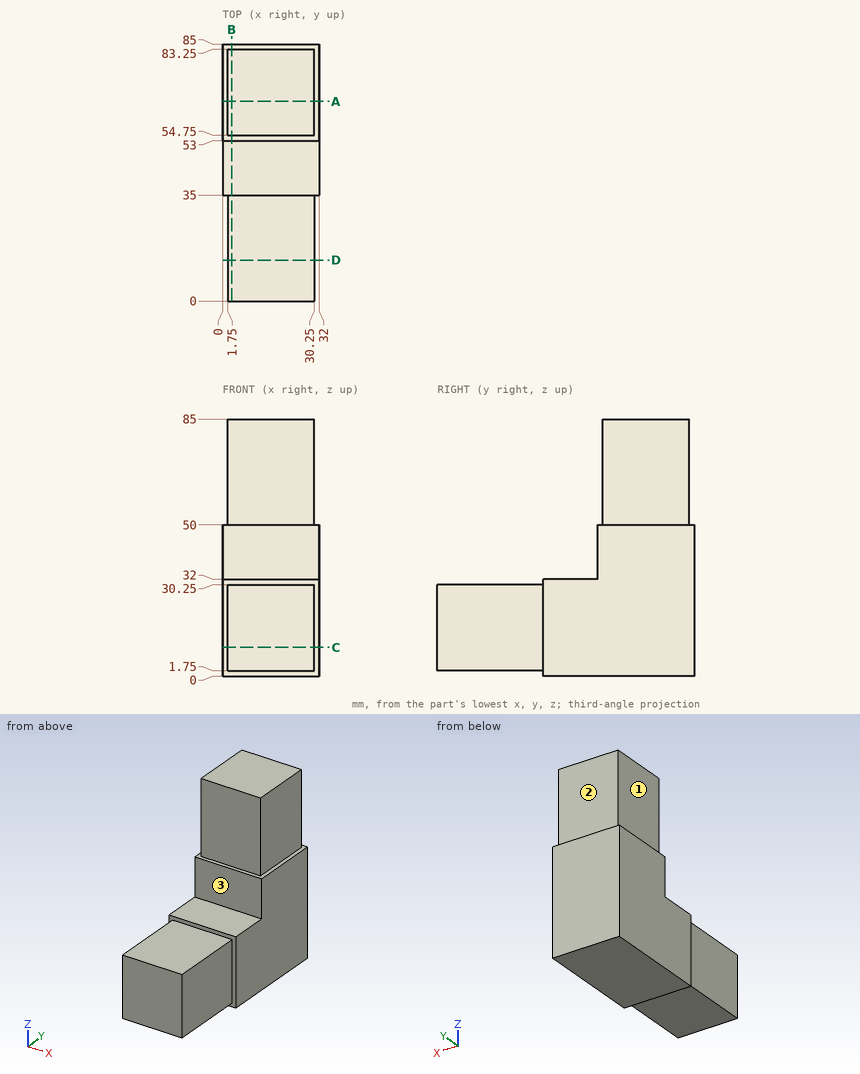
Verification items for this drawing (mm, ordinates from the low corner). A direction names the side the tool comes from. Coordinates: 2 decimals unless noted, no trailing zeros. Order: outer loops, then holes, each group sorted by start corner. A loop starts at its lowest first (then second) coordinate and runs counter-clockwise, first axis right, second up. Notation, with made-up numbers: (89.25, 57) - (130.25, 57) arc R20 ccw to (130.25, 84) - close; hole circle Ø1 at (-39.5, -13). An arc over 180 degrees is marked (long way). Use one line per item in the form item = value.
1. Access from +Z, -Z, +X, -X, +Y, -Y to the whole of each face (thin tool, end or side, straight path). Record for the marked faces 1, 2 and 3.
Here are the results:
face_1 = +Z, -X, +Y, -Y
face_2 = +Z, +X, -X, +Y
face_3 = +Z, +X, -X, -Y
2. Gauge pin test, flat ends, axial feed: pin 1 (8.5 mm diameter, centred on y = 25, z = 15.5, fed in from -X); pin 2 (9 mm diameter, centred on x = 16, z = 38.5, fed in from -Y); pin 3 (4 mm diameter, centred on x = 19, y = 45.5, fed in from +Z); pin 4 (4 mm diameter, centred on y = 36, z = 32, fed in from -X). Record the tip position at first contact, or that the pin passes through.
Here are the results:
pin_1 = 1.75
pin_2 = 53
pin_3 = 32
pin_4 = 0
3. Section check B-B (x = 3). Record the boundary of the cut face in (y, z).
Here are the results:
outline = (0, 1.75) - (35, 1.75) - (35, 0) - (85, 0) - (85, 50) - (83.25, 50) - (83.25, 85) - (54.75, 85) - (54.75, 50) - (53, 50) - (53, 32) - (35, 32) - (35, 30.25) - (0, 30.25) - close
4. Section check D-D (y = 13.5). Record the boundary of the cut face in (x, z), then the cut area to 3 significant figures.
Here are the results:
outline = (1.75, 1.75) - (30.25, 1.75) - (30.25, 30.25) - (1.75, 30.25) - close
area = 812 mm²
5. Scan lines: line 1 (Z direction, x = 6, y = 10); line 2 (Y direction, x = 29, z = 49); line 3 (Z direction, x = 20.5, y = 37.5). Record each from-to range of solid material in increasing order.
Here are the results:
line_1 = 1.75 to 30.25
line_2 = 53 to 85
line_3 = 0 to 32
6. Section check C-C (z = 9.5). Record the boundary of the cut face in (x, y), then the cut area to 3 significant figures.
Here are the results:
outline = (0, 35) - (1.75, 35) - (1.75, 0) - (30.25, 0) - (30.25, 35) - (32, 35) - (32, 85) - (0, 85) - close
area = 2,600 mm²
7. Section check A-A (y = 66). Record the boundary of the cut face in (x, z), then the cut area to 3 significant figures.
Here are the results:
outline = (0, 0) - (32, 0) - (32, 50) - (30.25, 50) - (30.25, 85) - (1.75, 85) - (1.75, 50) - (0, 50) - close
area = 2,600 mm²
